```python
from build123d import *

# Parameters (mm, degrees)
BOSS_EXTRUDE1_DEPTH      = 1
BOSS_EXTRUDE1_DEPTH_BACK = 2.5
BOSS_EXTRUDE2_DEPTH      = 0.5
BOSS_EXTRUDE2_DEPTH_BACK = 2.5
SKETCH4_W                = 0.5
SKETCH4_H                = 0.5
CUT_EXTRUDE1_DEPTH       = 12.250925888


with BuildPart() as part:
    # Sketch1 → Boss-Extrude1 (new, two sides: drawn at the far end of the back side and taken through both)
    with BuildSketch(Plane.XY.offset(-BOSS_EXTRUDE1_DEPTH_BACK)):
        Polygon((8.082903769, 0), (4.041451884, 7), (-4.041451884, 7), (-8.082903769, 0), (-4.041451884, -7), (4.041451884, -7), align=None)
        Polygon((6.581793069, 0), (3.290896534, 5.7), (-3.290896534, 5.7), (-6.581793069, 0), (-3.290896534, -5.7), (3.290896534, -5.7), align=None, mode=Mode.SUBTRACT)
    extrude(amount=BOSS_EXTRUDE1_DEPTH + BOSS_EXTRUDE1_DEPTH_BACK)

    # Sketch3 → Boss-Extrude2 (add, two sides: drawn at the far end of the back side and taken through both)
    with BuildSketch(Plane.XY.offset(-BOSS_EXTRUDE2_DEPTH_BACK)):
        Polygon((6.581793069, 0), (3.290896534, 5.7), (-3.290896534, 5.7), (-6.581793069, 0), (-3.290896534, -5.7), (3.290896534, -5.7), align=None)
        Polygon((6.119912853, 0), (3.059956427, 5.3), (-3.059956427, 5.3), (-6.119912853, 0), (-3.059956427, -5.3), (3.059956427, -5.3), align=None, mode=Mode.SUBTRACT)
    extrude(amount=BOSS_EXTRUDE2_DEPTH + BOSS_EXTRUDE2_DEPTH_BACK)

    # Sketch4 → Cut-Extrude1 (cut, through all)
    with BuildSketch(Plane.XY.offset(1)):
        with Locations((-1.224779595, 6.75)):
            Rectangle(SKETCH4_W, SKETCH4_H)
        with Locations((-0.224779595, 6.75)):
            Rectangle(SKETCH4_W, SKETCH4_H)
    extrude(amount=-CUT_EXTRUDE1_DEPTH, mode=Mode.SUBTRACT)


solid = part.part
```
Geometry: final body of the model. Coordinates: model frame, mm. A direction names the side the tool comes from. Coordinates: 2 decimals unless noted, no trailing zeros. Loops run counter-clockwise (first coordinate to the right, second up) from the corner with the lowest first, then second, coordinate; pieces in that order, holes last. Notation, with made-up numbers: (62, 1.5) -> (120, 1.5) arc R29 ccw to (120, 24.5) -> close; hole circle Ø2 at (78, -16). An arc over 180 degrees is marked (long way). Use a Markdown table: item, result. Add a question column.
(1) Mould query, pull axis Y, two halves, no side actions, for faces 1 (the flat face through (-4.611, -2.613, -1.021)), 2 (the flat face through (0, 6, 1)), 3 (the flat face through (0, -7, -1)). Classes: pulls with the +Y half, pulls with the -Y half, needs draft (parallel to the pull), parting line crosses it, or undercut.
(2) Line query: line 1 along Y through (x, z) = (-0.25, -0.9); line 2 along Y through (x, z) = (2, 0.6); line 3 along X through (y, z) = (2.5, -2.15). Output: solid intervals per line, ascending.
(3) Section query B-B, the plane x = 2. Return loops of the section in (y, z), plus the area to 3 significant figures.
(4) Section query D-D, the plane x = -7. Return loops of the section in (y, z).
(5) Section query C-C, the plane y = 1. Return loops of the section in (x, z).
(6) Section query A-A, the plane z = 0.8. Return loops of the section in (x, y).
(7) Access query for faces 4 (the flat face through (0, 5.3, -1)), 5 (the flat face through (4.8, 2.6, 0.5)), 6 (the flat face through (-3, 7, -1)). Directions: +Z, -Z, +X, -X, +Y, -Y. A direction counts if a zero-diameter tool reaches every point of the face in a straight line with its end or side. Return the directions, or none.
(8) Pin query (flat end, axial travel): pin 1 Ø0.6 at (y, z) = (6.5, -1.5) entering from +X; pin 2 Ø0.6 at (y, z) = (6.5, -1.5) entering from -X; pin 3 Ø1 at (y, z) = (-2, -0.5) entering from -X. Return the tip coordinate at first contact, or that it passes through.
Answer:
| question | item | result |
|---|---|---|
| 1 | face 1 | undercut |
| 1 | face 2 | needs draft |
| 1 | face 3 | pulls with the -Y half |
| 2 | line 1 | y = -7 to -5.3, 5.3 to 6.5 |
| 2 | line 2 | y = -7 to -5.7, 5.7 to 7 |
| 2 | line 3 | x = -6.64 to -4.68, 4.68 to 6.64 |
| 3 | outline | (-7, -2.5) -> (-5.3, -2.5) -> (-5.3, 0.5) -> (-5.7, 0.5) -> (-5.7, 1) -> (-7, 1) -> close; (5.3, -2.5) -> (7, -2.5) -> (7, 1) -> (5.7, 1) -> (5.7, 0.5) -> (5.3, 0.5) -> close |
| 3 | area | 11.5 mm^2 |
| 4 | outline | (-1.88, -2.5) -> (1.88, -2.5) -> (1.88, 1) -> (-1.88, 1) -> close |
| 5 | outline | (-7.51, -2.5) -> (-5.54, -2.5) -> (-5.54, 0.5) -> (-6, 0.5) -> (-6, 1) -> (-7.51, 1) -> close; (5.54, -2.5) -> (7.51, -2.5) -> (7.51, 1) -> (6, 1) -> (6, 0.5) -> (5.54, 0.5) -> close |
| 6 | outline | (-8.08, 0) -> (-4.04, -7) -> (4.04, -7) -> (8.08, 0) -> (4.04, 7) -> (0.03, 7) -> (0.03, 6.5) -> (-0.47, 6.5) -> (-0.47, 7) -> (-0.97, 7) -> (-0.97, 6.5) -> (-1.47, 6.5) -> (-1.47, 7) -> (-4.04, 7) -> close; hole (-6.58, 0) -> (-3.29, -5.7) -> (3.29, -5.7) -> (6.58, 0) -> (3.29, 5.7) -> (-3.29, 5.7) -> close |
| 7 | face 4 | +Z, -Z |
| 7 | face 5 | +Z |
| 7 | face 6 | +Z, -Z, +X, -X, +Y |
| 8 | pin 1 | stops at x = 4.5 |
| 8 | pin 2 | stops at x = -4.5 |
| 8 | pin 3 | stops at x = -7.22 |
